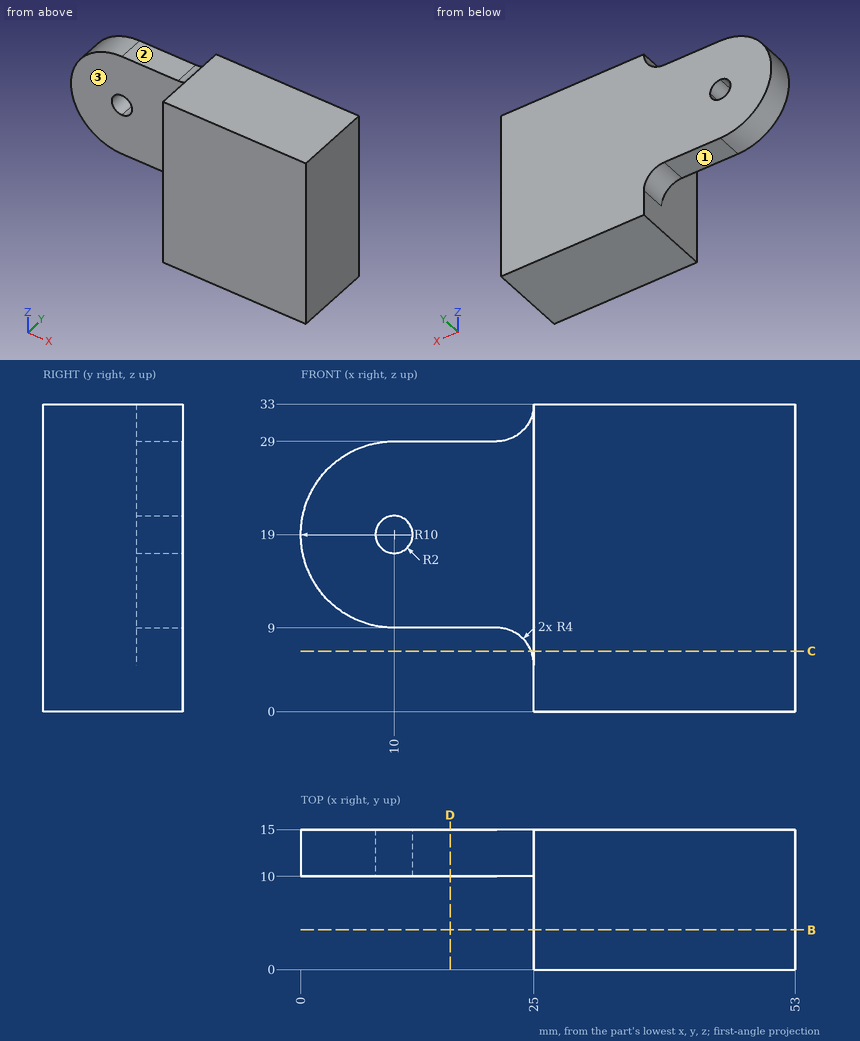
Drawing for the job (mm, zero at the part's lowest x, y, z). A direction names the side the tool comes from. Coordinates: 2 decimals unless noted, no trailing zeros. Write each loop counter-clockwise with the first axis right and the second up, starting at its lowest first coordinate (ties: lowest second). Pieces come first, ordered by that corner, then holes. Notation, with made-up numbers: (11, 37) - (18, 37) arc R14 ccw to (18, 55) - close; hole circle Ø4 at (19.5, 9.25). An arc over 180 degrees is marked (long way). Write each question's results on one line, items separated by ' | '. Start each with the question number.
1) Cut at D-D (x = 16). Write the cut outline in (y, z), then the cut area to 3 significant figures.
2) Cut at C-C (z = 6.5). Write the cut outline in (x, y).
3) Cut at B-B (y = 4.25). Write the cut outline in (x, z), then the cut area to 3 significant figures.
4) 3-axis set-ups, long thin cutter, end or side, ignore diameter. For the marked faces 1, 2 and 3: which of +Z, -Z, +X, -X, +Y, -Y reach the whole face in a straight line?
5) Flat gauge pins, fed straight in: P1, Ø6, axis at x = 26, z = 23.5, coming from the -Y side; P2, Ø12, axis at x = 8.5, z = 26.5, coming from the -Y side; P3, Ø1.5, axis at x = 16, y = 12, coming from the +Z side; P4, Ø2.5, axis at x = 17, y = 11.5, coming from the -Z side. Where does each tip first touch, or does it go through?
6) Probe line 1 along X through (y, z) = (8.75, 22.5); line 2 along Y through (x, z) = (19, 18.5); line 3 along X through (y, z) = (14.75, 19). List the from-to ranges inside material, lowest first. Write a range as from..to.
Returned:
1) outline: (10, 9) - (15, 9) - (15, 29) - (10, 29) - close | area: 100 mm^2
2) outline: (24.71, 10) - (25, 10) - (25, 0) - (53, 0) - (53, 15) - (24.71, 15) - close
3) outline: (25, 0) - (53, 0) - (53, 33) - (25, 33) - close | area: 924 mm^2
4) face 1: -Z, -X, +Y, -Y | face 2: +Z, -X, +Y, -Y | face 3: +Z, -Z, -X, -Y
5) P1: y = 0 | P2: y = 10 | P3: z = 29 | P4: z = 9
6) line 1: 25..53 | line 2: 10..15 | line 3: 0..8, 12..53
